```python
from build123d import *

# Parameters (mm, degrees)
CIRPATTERN1_COUNT = 3


with BuildPart() as part:
    # Sketch1 → Revolve1 (revolve)
    with BuildSketch(Plane.XY):
        with BuildLine():
            Line((0, 3.85), (0, 1.5))
            Line((0, 1.5), (5.711324865, 1.5))
            Line((5.711324865, 1.5), (6, 1))
            Line((6, 1), (6, 0))
            Line((6, 0), (-10, 0))
            ThreePointArc((-10, 0), (-9.952671274, 0.212341041), (-9.819645129, 0.384482759))
            ThreePointArc((-9.819645129, 0.384482759), (-5.328465382, 2.957041529), (-0.230291267, 3.85))
            Line((-0.230291267, 3.85), (0, 3.85))
        make_face()
    revolve(axis=Axis((-88.99, 0, 0), (1, 0, 0)))

    # Sketch5 → Ø1.0mm Dowel Hole1 (revolve, cut)
    with BuildSketch(Plane(origin=(0, 2.65, 0), x_dir=(0, 0, -1), z_dir=(0, 1, 0))):
        Polygon((0, 0), (0, 8.80043031), (0.5, 8.5), (0.5, 0), align=None)
    f_1_0mm_dowel_hole1 = revolve(axis=Axis((6.35, 2.65, 0), (-1, 0, 0)), mode=Mode.SUBTRACT)

    # CirPattern1: Ø1.0mm Dowel Hole1 ×3 about axis
    cirpattern1_axis = Axis((0, 0, 0), (1, 0, 0))
    for i in range(1, CIRPATTERN1_COUNT):
        add(f_1_0mm_dowel_hole1.rotate(cirpattern1_axis, i * 360 / CIRPATTERN1_COUNT), mode=Mode.SUBTRACT)


solid = part.part
```
Could you check a few things on this model? Use its own coordinates, in mm. Coordinates: 2 decimals unless noted, no trailing zeros. Write each loop counter-clockwise with the first axis right and the second up, starting at its lowest first coordinate (ties: lowest second). Pieces come first, ordered by that corner, then holes. Notation, with made-up numbers: (-3, 78.5) - (51, 78.5) arc R25 cw to (51, 102.5) - close; hole circle Ø8 at (23, 22). An arc over 180 degrees is marked (long way). Use a Markdown table: item, result.
Q1. Thinking about a two-plate mould opening in Y: for faces 1 (the flat face through (0, 1.7, 0.1)), 2 (the cylindrical face through (-2.737, -1.133, 1.833)), 3 (the cylindrical face through (2.9, -1.5, 0.07)), which applies, +Y half, -Y half, draft (parallel to the pull), parting line (faces both ways), or undercut?
Geometry check:
| item | result |
|---|---|
| face 1 | draft |
| face 2 | undercut |
| face 3 | parting line |
Q2. I'm going to push flat-ended pins straight in: pin 1 Ø4 at (x, z) = (-6, 1.5) entering from -Y; pin 2 Ø3 at (y, z) = (-2.5, -1) entering from -X; pin 3 Ø2 at (y, z) = (-2, -0.5) entering from -X. Where does each tip first touch, or does it pass through?
Geometry check:
| item | result |
|---|---|
| pin 1 | stops at y = -3.26 |
| pin 2 | stops at x = -8.75 |
| pin 3 | stops at x = -8.94 |
Q3. Please list where these lines run through material, in increasing order: L1, parallel to Z at x = -1, y = -1.75; L2, parallel to Z at x = -6.25, y = 2.25; L3, parallel to Y at x = -2.75, z = 2.
Geometry check:
| item | result |
|---|---|
| L1 | z = -3.41 to -2.56, -2.03 to 2.03, 2.56 to 3.41 |
| L2 | z = -1.28 to -0.3, 0.3 to 1.28 |
| L3 | y = -3.04 to -1.73, -0.92 to 3.04 |
Q4. Imagine slicing it at A-A (x = 1.75). List the corners of the cut face in (y, z) for me.
Geometry check:
| item | result |
|---|---|
| outline | circle Ø3 at (0, 0) |
